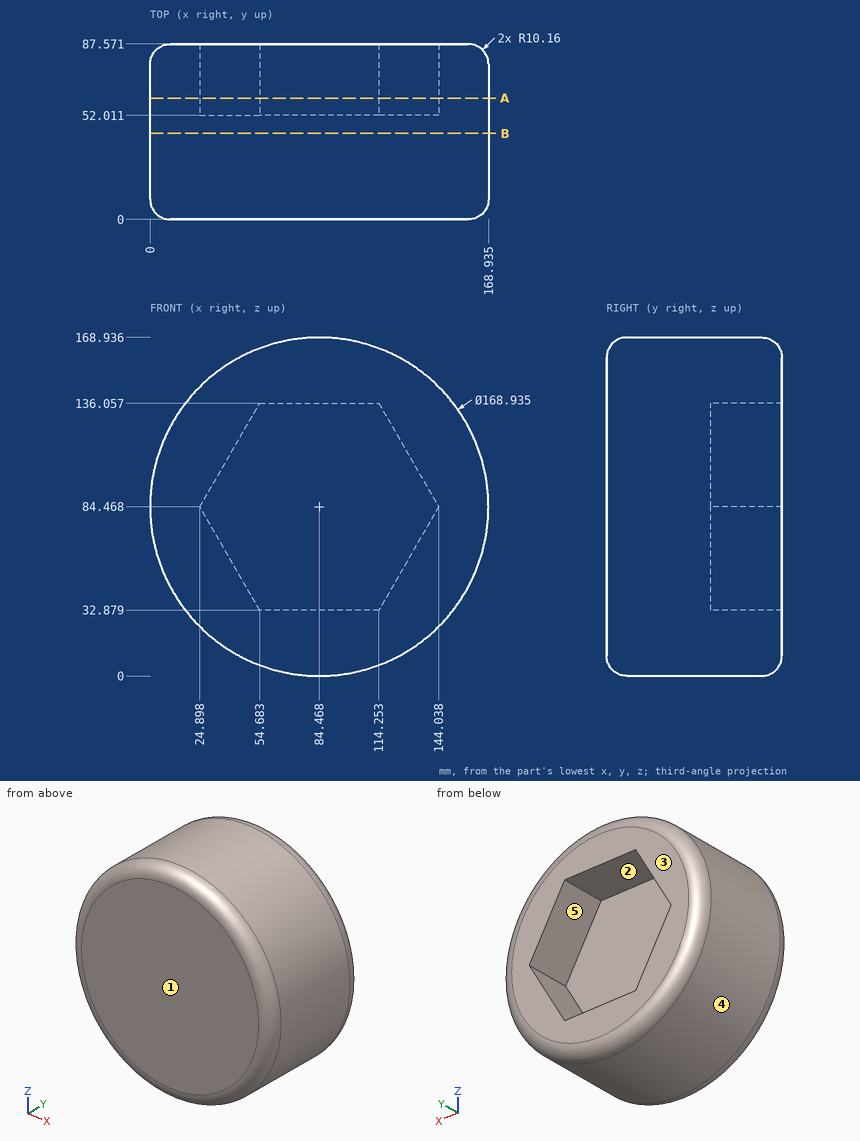
Here's the drawing with two shaded views (mm, measured from the low corner). I have some questions. A direction names the side the tool comes from. Round coordinates to 2 decimals unless told otherwise and drop trailing zeros. Order: outer loops, then holes, each group sorted by start corner. A loop starts at its lowest first (then second) coordinate and runs counter-clockwise, first axis right, second up. Notation, with made-up numbers: M 8,66.25 L 29,66.25 A19 ccw 29,95.25 Z; hole C -20.75,-10 d1. An arc over 180 degrees is marked long. Use CSV: the item, a comma, the result in double quotes.
1) I need wall thicknesses on line 1 along Y through (x, z) = (73, 101); line 2 along X through (y, z) = (74, 49) (1 decimal); line 3 along X through (y, z) = (77.5, 123) (1 decimal). Which ranges of each line are inside material? Lowest first, please. Write a range as [from, to].
Taken from the geometry:
line 1,"[0, 52.01]"
line 2,"[7.8, 45.4], [123.6, 161.1]"
line 3,"[9.3, 47.1], [121.8, 159.6]"
2) On a 3-axis mill with a long thin cutter (end or side, diameter ignored), from which of +Z, -Z, +X, -X, +Y, -Y can I reach the whole of each face in a straight line? I mean the marked faces 1 and 2. Say none if no direction works.
Taken from the geometry:
face 1,"+Z, -Z, +X, -X, -Y"
face 2,"+Y"
3) I'm going to push flat-ended pins straight in: P1, Ø1.5, axis at y = 77, z = 101.5, coming from the +X side; P2, Ø1.5, axis at x = 69, z = 33, coming from the +Y side; P3, Ø1.5, axis at x = 112.5, y = 66.5, coming from the -Z side; P4, Ø1.5, axis at y = 65.5, z = 41.5, coming from the -X side. Where does each tip first touch, or does it pass through?
Taken from the geometry:
P1,"x = 167.35"
P2,"y = 87.57"
P3,"z = 4.53"
P4,"x = 11.31"
4) I want a section at A-A (y = 60.5). List the corners of the cut face in (x, z) for me (1 decimal).
Taken from the geometry:
outline,"C 84.5,84.5 d168.9; hole M 24.9,84.5 L 54.7,32.9 L 114.3,32.9 L 144,84.5 L 114.3,136.1 L 54.7,136.1 Z"
5) If we mould it in two halves opening along Z, with no side actions, what happens to the marked faces 3, 4 and 5? For each: pulls with the +Z half, pulls with the -Z half, needs draft (parallel to the pull), parting line crosses it, or undercut.
Taken from the geometry:
face 3,"needs draft"
face 4,"parting line crosses it"
face 5,"undercut"
6) I want a section at B-B (y = 43). List the corners of the cut face in (x, z) for me (1 decimal), then the cut area to 3 significant figures.
Taken from the geometry:
outline,"C 84.5,84.5 d168.9"
area,"22,400 mm^2"
